Source: CAD feature listing. Evaluate the final solid. Frame: model axes, mm. Round coordinates to 2 decimals unless told otherwise and drop trailing zeros. Write each loop counter-clockwise with the first axis right and the second up, starting at its lowest first coordinate (ties: lowest second). Pieces come first, ordered by that corner, then holes. Notation, with made-up numbers: M 23.25,-9.75 L 67.25,-9.75 A35 cw 67.25,23.25 Z; hole C -13,39 d9. An arc over 180 degrees is marked long. Answer in a Markdown table with one row per item. Add a question column.
Item 1: Cut plane C-C on x = -93.5. Give the number of separate pieces and of enclosed holes in the cut face, and give its area (3 significant figures).
Item 2: Material intervals for probe 1 along Y at (x, z) = (-93.75, 3.5); probe 2 along Y at (x, z) = (-93.5, -32); probe 3 along Z at (x, y) = (-90, 1), sorted ascending.
Item 3: Cut plane D-D on z = -26.5. Return loops of the section in (x, y).
Item 4: Cut plane A-A on z = 0. Return loops of the section in (x, y) (3 decimals).
Item 5: Contact query for a flat-ended pin moving along its axis: pin 1 (1.5 mm diameter, centred on x = -94.5, y = -26.5, fed in from +Z). Output: stop coordinate, or through.
Item 6: Cut plane B-B on y = -24. Return loops of the section in (x, z), and give its area (3 significant figures).
Item 7: Mould query, pull axis Y, two halves, no side actions, for faces 1 (the face through (-92.031, -36.053, -34.49)), 2 (the face through (-92.03, -32.77, -42.73)), 3 (the face through (-88.9, 0.8, 35.1)). Classes: released by +Y, released by -Y, zero draft, split by the parting line, or undercut.
from build123d import *

# Parameters (mm, degrees)
SKETCH1_R           = 53.848
SKETCH1_R_2         = 34.925
SKETCH1_R_3         = 2.4892
BOSS_EXTRUDE1_DEPTH = 6.35


with BuildPart() as part:
    # Sketch1 → Boss-Extrude1 (new body)
    with BuildSketch(Plane.ZY.offset(88.9)):
        Circle(SKETCH1_R)
        Circle(SKETCH1_R_2, mode=Mode.SUBTRACT)
        with Locations((-33.845113149, 35.638918571)):
            Circle(SKETCH1_R_3, mode=Mode.SUBTRACT)
        with Locations((1.268411978, 49.132630014)):
            Circle(SKETCH1_R_3, mode=Mode.SUBTRACT)
        with Locations((35.638918571, 33.845113149)):
            Circle(SKETCH1_R_3, mode=Mode.SUBTRACT)
        with Locations((49.132630014, -1.268411978)):
            Circle(SKETCH1_R_3, mode=Mode.SUBTRACT)
        with Locations((33.845113149, -35.638918571)):
            Circle(SKETCH1_R_3, mode=Mode.SUBTRACT)
        with Locations((-1.268411978, -49.132630014)):
            Circle(SKETCH1_R_3, mode=Mode.SUBTRACT)
        with Locations((-35.638918571, -33.845113149)):
            Circle(SKETCH1_R_3, mode=Mode.SUBTRACT)
        with Locations((-49.132630014, 1.268411978)):
            Circle(SKETCH1_R_3, mode=Mode.SUBTRACT)
    extrude(amount=BOSS_EXTRUDE1_DEPTH)


solid = part.part
Results below:
| question | item | result |
|---|---|---|
| 1 | separate pieces | 1 |
| 1 | enclosed holes | 9 |
| 1 | area | 5,120 mm2 |
| 2 | probe 1 | -53.73 to -34.75, 34.75 to 48.03, 50.24 to 53.73 |
| 2 | probe 2 | -43.31 to -13.99, 13.99 to 33.97, 37.31 to 43.31 |
| 2 | probe 3 | -53.84 to -51.61, -46.66 to -34.91, 34.91 to 48.11, 50.16 to 53.84 |
| 3 | outline | M -95.25,-46.88 L -88.9,-46.88 L -88.9,-22.75 L -95.25,-22.75 Z; M -95.25,22.75 L -88.9,22.75 L -88.9,46.88 L -95.25,46.88 Z |
| 4 | outline | M -95.25,-53.848 L -88.9,-53.848 L -88.9,-51.274 L -95.25,-51.274 Z; M -95.25,-46.991 L -88.9,-46.991 L -88.9,-34.925 L -95.25,-34.925 Z; M -95.25,34.925 L -88.9,34.925 L -88.9,46.991 L -95.25,46.991 Z; M -95.25,51.274 L -88.9,51.274 L -88.9,53.848 L -95.25,53.848 Z |
| 5 | pin 1 | z = 47.29 |
| 6 | outline | M -95.25,-48.2 L -88.9,-48.2 L -88.9,-25.37 L -95.25,-25.37 Z; M -95.25,25.37 L -88.9,25.37 L -88.9,48.2 L -95.25,48.2 Z |
| 6 | area | 290 mm2 |
| 7 | face 1 | undercut |
| 7 | face 2 | split by the parting line |
| 7 | face 3 | zero draft |
